Could you check a few things on this model? Use its own coordinates, in mm. Face numbers are marked on the shaded views. A direction names the side the tool comes from. Give positions to 0.01 mm unless a question says otherwise; leave off trailing zeros. Order: outer loops, then holes, each group sorted by start corner. A loop starts at its lowest first (then second) coordinate and runs counter-clockwise, first axis right, second up. Notation, with made-up numbers: M -32,18.25 L 15,18.25 A16 ccw 15,37.25 Z; hole C -34,84 d5. An arc over 180 degrees is marked long. Use a Markdown table: item, result. Add a question column.
Item 1: Suppose I cut it at C-C on x = 0. Write out the boundary of the cut face in (y, z) (3 decimals), plus the area to 3 significant figures.
Item 2: Suppose I cut it at A-A on y = 24.5. Write out the boundary of the cut face in (x, z) (3 decimals).
Item 3: I'm going to push flat-ended pins straight in: pin 1 Ø8 at (x, z) = (-3.5, 8.5) entering from -Y; pin 2 Ø1.9 at (y, z) = (72, 8) entering from +X; pin 3 Ø16 at (x, y) = (-30.5, 31) entering from -Z; pin 4 Ø10 at (x, z) = (-32, 49.5) entering from -Y. Where does each tip first touch, or does it pass through?
Item 4: If I drill on L1, parallel to X at y = 36.5, z = 53.5; L2, parallel to X at y = 34.5, z = 45.5; L3, parallel to Z at x = -27, y = 65 (3 decimals), over which ranges is the centre line in solid material (lowest first)? Write a range as from..to.
Item 5: If we mould it in two halves opening along X, with no side actions, what happens to the marked faces 5, 6 and 7? For each: released by +X, released by -X, zero draft, split by the parting line, or undercut.
Item 6: Suppose I cut it at D-D on z = 54. Write out the boundary of the cut face in (x, y), plus the area to 3 significant figures.
Item 7: Suppose I cut it at B-B on z = 44. Write out the boundary of the cut face in (x, y).
Item 8: For the marked faces 1, 2, 3 and 4, which set-ups out of +Z, -Z, +X, -X, +Y, -Y let a thin tool reach every point of the face, with its end or its side?
Autodesk Fusion 360 part; units mm, degrees
sketch "Sketch1" plane through (0, 0, 0) normal (0, 1, 0) x (1, 0, 0)
  circle A0 centre (0, 0) radius 7.7724
  dimension "d1" = 15.5448
extrude "Extrude1" add sketch "Sketch1" along normal blind 76.2
sketch "Sketch2" plane through (0, 76.2, 0) normal (0, 1, 0) x (-1, 0, 0)
  circle A0 centre (0, 0) radius 7.7724
  line L0 (-7.7723, 0.0299) -> (7.7725, 0.0299)
  line L1 (7.7725, 0.0299) -> (7.7725, 17.6304)
  line L2 (7.7725, 17.6304) -> (-7.7723, 17.6304)
  line L3 (-7.7723, 17.6304) -> (-7.7723, 0.0299)
  dimension "d4" = 15.5448
extrude "Extrude2" add sketch "Sketch2" against normal blind 6.35 contours A0 L1 L2 L3
sketch "Sketch3" plane through (0, 0, 17.6304) normal (0, 0, 1) x (-1, 0, 0)
  line L0 (-7.7723, -76.2) -> (7.7725, -76.2)
  line L1 (7.7725, -76.2) -> (7.7725, -69.85)
  line L2 (7.7725, -69.85) -> (-7.7723, -69.85)
  line L3 (-7.7723, -69.85) -> (-7.7723, -76.2)
  line L4 (-50.8, -76.2) -> (50.8, -76.2)
  line L5 (50.8, -76.2) -> (50.8, -12.7)
  line L6 (50.8, -12.7) -> (-50.8, -12.7)
  line L7 (-50.8, -12.7) -> (-50.8, -76.2)
  dimension "d7" = 101.6
  dimension "d8" = 63.5
extrude "Extrude3" add sketch "Sketch3" along normal blind 21.5646
sketch "Sketch4" plane through (0, 0, 39.195) normal (0, 0, 1) x (-1, 0, 0)
  line L0 (-50.8, -12.7) -> (-50.8, -76.2)
  line L1 (-50.8, -76.2) -> (50.8, -76.2)
  line L2 (50.8, -76.2) -> (50.8, -12.7)
  line L3 (50.8, -12.7) -> (-50.8, -12.7)
  line L4 (50.8, -12.7) -> (41.91, -12.7)
  line L5 (41.91, -12.7) -> (41.91, -76.2)
  line L6 (41.91, -76.2) -> (50.8, -76.2)
  line L7 (50.8, -76.2) -> (50.8, -12.7)
  line L8 (-50.8, -76.2) -> (-41.91, -76.2)
  line L9 (-41.91, -76.2) -> (-41.91, -12.7)
  line L10 (-41.91, -12.7) -> (-50.8, -12.7)
  line L11 (-50.8, -12.7) -> (-50.8, -76.2)
  dimension "d11" = 8.89
  dimension "d12" = 63.5
  dimension "d13" = 8.89
extrude "Extrude4" add sketch "Sketch4" along normal blind 20.32 contours L0 L1 L3 L8 L9 L10 L11 | L1 L2 L3 L4 L5 L6 L7
sketch "Sketch5" plane through (-41.91, 0, 0) normal (1, 0, 0) x (0, 1, 0)
  line L0 (12.7, 39.195) -> (76.2, 39.195)
  line L1 (76.2, 39.195) -> (76.2, 59.515)
  line L2 (76.2, 59.515) -> (12.7, 59.515)
  line L3 (12.7, 59.515) -> (12.7, 39.195)
  line L4 (12.7, 59.515) -> (76.2, 59.515)
  line L5 (76.2, 59.515) -> (76.2, 54.435)
  line L6 (76.2, 54.435) -> (12.7, 54.435)
  line L7 (12.7, 54.435) -> (12.7, 59.515)
  dimension "d16" = 63.5
  dimension "d17" = 5.08
sketch "Sketch6" plane through (41.91, 0, 0) normal (-1, 0, 0) x (0, -1, 0)
  line L0 (-76.2, 39.195) -> (-12.7, 39.195)
  line L1 (-12.7, 39.195) -> (-12.7, 59.515)
  line L2 (-12.7, 59.515) -> (-76.2, 59.515)
  line L3 (-76.2, 59.515) -> (-76.2, 39.195)
  line L4 (-76.2, 59.515) -> (-12.7, 59.515)
  line L5 (-12.7, 59.515) -> (-12.7, 54.435)
  line L6 (-12.7, 54.435) -> (-76.2, 54.435)
  line L7 (-76.2, 54.435) -> (-76.2, 59.515)
  dimension "d18" = 63.5
  dimension "d19" = 5.08
extrude "Extrude5" add sketch "Sketch5" along normal blind 31.75 contours L1 L2 L3 L4 L5 L6 L7
sketch "Sketch7" plane through (41.91, 0, 0) normal (-1, 0, 0) x (0, -1, 0)
extrude "Extrude6" add sketch "Sketch6" along normal blind 31.75 contours L1 L2 L3 L4 L5 L6 L7
extrude "Extrude7" cut 1 faces at (2.5908, 33.8667, 39.195) along direction (0, 0, -1) blind 7.62
extrude "Extrude8" add 2 faces at (-31.3267, 55.0333, 54.435) (31.3267, 33.8667, 54.435) along direction (0, 0, -1) blind 7.62
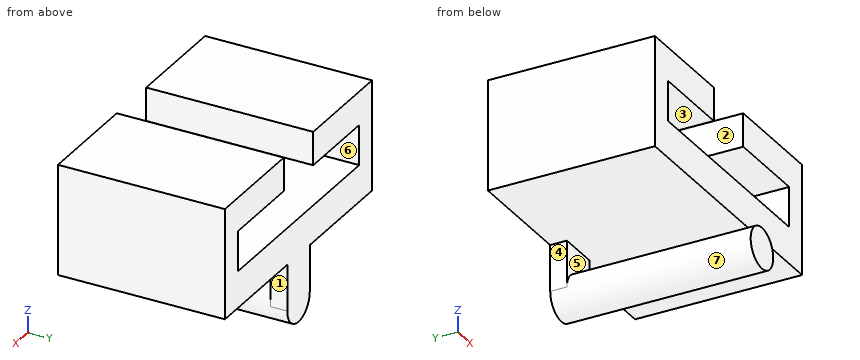
Findings below:
| question | item | result |
|---|---|---|
| 1 | outline | M 0,-7.772 L 76.2,-7.772 L 76.2,31.575 L 12.7,31.575 L 12.7,17.63 L 69.85,17.63 L 69.85,7.772 L 0,7.772 Z |
| 1 | area | 2,130 mm^2 |
| 2 | outline | M -50.8,17.63 L 50.8,17.63 L 50.8,59.515 L 10.16,59.515 L 10.16,46.815 L 41.91,46.815 L 41.91,31.575 L -41.91,31.575 L -41.91,46.815 L -10.16,46.815 L -10.16,59.515 L -50.8,59.515 Z; C 0,0 d15.545 |
| 3 | pin 1 | stops at y = 0 |
| 3 | pin 2 | stops at x = 7.77 |
| 3 | pin 3 | stops at z = 17.63 |
| 3 | pin 4 | stops at y = 12.7 |
| 4 | L1 | x = -50.8..-10.16, 10.16..50.8 |
| 4 | L2 | x = -50.8..-41.91, 41.91..50.8 |
| 4 | L3 | z = 17.63..31.575, 46.815..59.515 |
| 5 | face 5 | zero draft |
| 5 | face 6 | undercut |
| 5 | face 7 | split by the parting line |
| 6 | outline | M -50.8,12.7 L -10.16,12.7 L -10.16,76.2 L -50.8,76.2 Z; M 10.16,12.7 L 50.8,12.7 L 50.8,76.2 L 10.16,76.2 Z |
| 6 | area | 5,160 mm^2 |
| 7 | outline | M -50.8,12.7 L -41.91,12.7 L -41.91,76.2 L -50.8,76.2 Z; M 41.91,12.7 L 50.8,12.7 L 50.8,76.2 L 41.91,76.2 Z |
| 8 | face 1 | -Z, +X, +Y, -Y |
| 8 | face 2 | +Z, +Y, -Y |
| 8 | face 3 | +Y, -Y |
| 8 | face 4 | -Z, -X, +Y, -Y |
